```python
from build123d import *

# Parameters (mm, degrees)
SKETCH1_W           = 12.5
SKETCH1_H           = 29
BOSS_EXTRUDE1_DEPTH = 15.7
SKETCH2_R           = 0.45
BOSS_EXTRUDE2_DEPTH = 3.8


with BuildPart() as part:
    # Sketch1 → Boss-Extrude1 (new body)
    with BuildSketch(Plane(origin=(0, 0, 0), x_dir=(1, 0, 0), z_dir=(0, 1, 0))):
        Rectangle(SKETCH1_W, SKETCH1_H)
    extrude(amount=BOSS_EXTRUDE1_DEPTH)

    # Sketch2 → Boss-Extrude2 (add)
    with BuildSketch(Plane(origin=(0, 0, 0), x_dir=(1, 0, 0), z_dir=(0, 1, 0))):
        with Locations(Location((-3.75, -13.04, 0), (0, 0, 270))):
            Circle(SKETCH2_R)
        with Locations(Location((-3.75, -8.04, 0), (0, 0, 270))):
            Circle(SKETCH2_R)
        with Locations(Location((-3.75, -3.04, 0), (0, 0, 270))):
            Circle(SKETCH2_R)
        with Locations(Location((-3.75, 11.96, 0), (0, 0, 270))):
            Circle(SKETCH2_R)
        with Locations(Location((3.75, 11.96, 0), (0, 0, 90))):
            Circle(SKETCH2_R)
        with Locations(Location((3.75, -3.04, 0), (0, 0, 90))):
            Circle(SKETCH2_R)
        with Locations(Location((3.75, -8.04, 0), (0, 0, 90))):
            Circle(SKETCH2_R)
        with Locations(Location((3.75, -13.04, 0), (0, 0, 90))):
            Circle(SKETCH2_R)
    extrude(amount=-BOSS_EXTRUDE2_DEPTH)


solid = part.part
```
For this review, take the finished solid that the model builds, in its own axes (mm). A direction names the side the tool comes from. Round coordinates to 2 decimals unless told otherwise and drop trailing zeros. Loops run counter-clockwise (first coordinate to the right, second up) from the corner with the lowest first, then second, coordinate; pieces in that order, holes last.
Q1. To check wall thickness, follow line 1 along Y through (x, z) = (-4.5, -5). State the ranges of the line that lie inside material, in increasing order.
Result sheet:
line 1: y = 0 to 15.7
Q2. Add section A-A on x = -3.75. Write out the cut boundary in (y, z).
Result sheet:
outline: (-3.8, -12.41) - (0, -12.41) - (0, -14.5) - (15.7, -14.5) - (15.7, 14.5) - (0, 14.5) - (0, 13.49) - (-3.8, 13.49) - (-3.8, 12.59) - (0, 12.59) - (0, 8.49) - (-3.8, 8.49) - (-3.8, 7.59) - (0, 7.59) - (0, 3.49) - (-3.8, 3.49) - (-3.8, 2.59) - (0, 2.59) - (0, -11.51) - (-3.8, -11.51) - close
Q3. Add section C-C on z = 2. Write out the cut boundary in (x, y).
Result sheet:
outline: (-6.25, 0) - (6.25, 0) - (6.25, 15.7) - (-6.25, 15.7) - close
Q4. Machinability: for faces 1 (the face through (-3.73, -1.87, 7.59)), 2 (the face through (4, -3.8, 3)), which of the approach directions +Z, -Z, +X, -X, +Y, -Y give a long, thin tool a straight path to every point of the face, cutting with its end or side? Answer none if there is none.
Result sheet:
face 1: -Y
face 2: +Z, -Z, +X, -X, -Y
Q5. Mouldability with a two-part tool opening along Z and no side actions: class faces 3 (the face through (6.25, 8, 0)), 4 (the face through (-3.446, -1.873, 2.708)), 5 (the face through (0, 8, -14.5)) as +Z half, -Z half, draft (parallel to the pull), parting line (faces both ways), or undercut.
Result sheet:
face 3: draft
face 4: undercut
face 5: -Z half
Q6. Add section D-D on x = 1.25. Write out the cut boundary in (y, z).
Result sheet:
outline: (0, -14.5) - (15.7, -14.5) - (15.7, 14.5) - (0, 14.5) - close
Q7. Add section B-B on z = -11.96. Write out the cut boundary in (x, y), plus the area to 3 significant figures.
Result sheet:
outline: (-6.25, 0) - (-4.2, 0) - (-4.2, -3.8) - (-3.3, -3.8) - (-3.3, 0) - (3.3, 0) - (3.3, -3.8) - (4.2, -3.8) - (4.2, 0) - (6.25, 0) - (6.25, 15.7) - (-6.25, 15.7) - close
area: 203 mm2
